Can you work these out from the model? Positions are in its coordinate system, mm. Face numbers are marked on the shaded views. A direction names the side the tool comes from. Coordinates: 2 decimals unless noted, no trailing zeros. Order: outer loops, then holes, each group sorted by start corner. A loop starts at its lowest first (then second) coordinate and runs counter-clockwise, first axis right, second up. Notation, with made-up numbers: (27.5, 35.5) - (54.5, 35.5) arc R12 cw to (54.5, 56.5) - close; hole circle Ø10 at (-31, 75.25). An arc over 180 degrees is marked (long way). Use a Markdown table: item, result. Add a question column.
(1) I want a section at A-A (z = -11). List the corners of the cut face in (x, y) for me.
(2) If I drill on L1, parallel to Z at x = -0.75, y = 3; L2, parallel to X at y = 3, z = -1; L3, parallel to Z at x = 5.5, y = 9, over which ranges is the centre line in solid material (lowest first)? Write a range as [from, to].
(3) On a 3-axis mill with a long thin cutter (end or side, diameter ignored), from which of +Z, -Z, +X, -X, +Y, -Y can I reach the whole of each face in a straight line? I mean the marked faces 4, 5 and 6. Say none if no direction works.
(4) For pin 1 Ø4 at (y, z) = (-28, 11.5) entering from -X; pin 2 Ø4 at (y, z) = (-28, 16) entering from +X; pin 3 Ø1 at (x, z) = (3, 16.5) entering from +Y, each with a flat end and sliding along its axis, tell me the tip position at first contact or that it passes through.
(5) We'd pull the mould along Z, two halves only. Please class the marked faces 1, 2 and 3: pulls with the +Z half, pulls with the -Z half, needs draft (parallel to the pull), parting line crosses it, or undercut.
```python
from build123d import *

# Parameters (mm, degrees)
SKETCH1_W           = 10
SKETCH1_H           = 10
BOSS_EXTRUDE1_DEPTH = 10
SKETCH2_R           = 5
BOSS_EXTRUDE2_DEPTH = 10
SKETCH4_R           = 4
BOSS_EXTRUDE3_DEPTH = 40
BOSS_EXTRUDE4_DEPTH = 10
CUT_EXTRUDE1_DEPTH  = 10
FILLET2_R           = 5
SKETCH7_W           = 14
SKETCH7_H           = 14
BOSS_EXTRUDE5_DEPTH = 2


with BuildPart() as part:
    # Sketch1 → Boss-Extrude1 (new body)
    with BuildSketch(Plane(origin=(0, 0, 0), x_dir=(1, 0, 0), z_dir=(0, 1, 0))):
        with Locations((5, 5)):
            Rectangle(SKETCH1_W, SKETCH1_H)
    extrude(amount=BOSS_EXTRUDE1_DEPTH)

    # Sketch2 → Boss-Extrude2 (add)
    with BuildSketch(Plane(origin=(0, 0, -10), x_dir=(-1, 0, 0), z_dir=(0, 0, -1))):
        with Locations((-5, 5)):
            Circle(SKETCH2_R)
    extrude(amount=BOSS_EXTRUDE2_DEPTH)

    # Sketch4 → Boss-Extrude3 (add)
    with BuildSketch(Plane(origin=(9.62e-07, 9.026239035, -5.211301537), x_dir=(0, -0.49999999999999467, -0.8660254037844417), z_dir=(-9.225892847871432e-08, -0.8660254037844382, 0.4999999999999926))):
        with Locations(Location((2.59569937, 4.999999038, 0), (0, 0, 229.539411428))):
            Circle(SKETCH4_R)
    extrude(amount=BOSS_EXTRUDE3_DEPTH)

    # Sketch5 → Boss-Extrude4 (add)
    with BuildSketch(Plane(origin=(0, 0, 0), x_dir=(0, 0, -1), z_dir=(1, 0, 0))):
        with BuildLine():
            Line((-16.004858714, -24.912627201), (-9.076655484, -28.912627201))
            ThreePointArc((-9.076655484, -28.912627201), (-6.076655484, -34.108779624), (-9.076655484, -39.304932046))
            Line((-9.076655484, -39.304932046), (-12.71063008, -37.206855835))
            Line((-12.71063008, -37.206855835), (-10.21063008, -32.876728816))
            Line((-10.21063008, -32.876728816), (-18.870884118, -27.876728816))
            Line((-18.870884118, -27.876728816), (-21.370884118, -32.206855835))
            Line((-21.370884118, -32.206855835), (-25.004858714, -30.108779624))
            ThreePointArc((-25.004858714, -30.108779624), (-22.004858714, -24.912627201), (-16.004858714, -24.912627201))
        make_face()
    extrude(amount=BOSS_EXTRUDE4_DEPTH)

    # Sketch6 → Cut-Extrude1 (cut)
    with BuildSketch(Plane(origin=(0, -33.40900615, 19.288698694), x_dir=(-1, 0, 0), z_dir=(0, -0.8660254037844403, 0.4999999999999971))):
        with BuildLine():
            Line((0, -7.40430063), (0, -2.40430063))
            ThreePointArc((0, -2.40430063), (-1.464466094, -5.939834536), (-5, -7.40430063))
            Line((-5, -7.40430063), (0, -7.40430063))
        make_face()
        with BuildLine():
            Line((-10, -7.40430063), (-5, -7.40430063))
            ThreePointArc((-5, -7.40430063), (-8.535533906, -5.939834536), (-10, -2.40430063))
            Line((-10, -2.40430063), (-10, -7.40430063))
        make_face()
        with BuildLine():
            ThreePointArc((-7.718879336, 11.791851793), (-6.417610293, 12.390527944), (-5, 12.59569937))
            Line((-5, 12.59569937), (-10, 12.59569937))
            Line((-10, 12.59569937), (-10, 11.791851793))
            Line((-10, 11.791851793), (-7.718879336, 11.791851793))
        make_face()
        with BuildLine():
            ThreePointArc((-10, 7.59569937), (-9.392857651, 9.983753318), (-7.718879336, 11.791851793))
            Line((-7.718879336, 11.791851793), (-10, 11.791851793))
            Line((-10, 11.791851793), (-10, 7.59569937))
        make_face()
        with BuildLine():
            Line((-2.281120664, 11.791851793), (0, 11.791851793))
            Line((0, 11.791851793), (0, 12.59569937))
            Line((0, 12.59569937), (-5, 12.59569937))
            ThreePointArc((-5, 12.59569937), (-3.582389707, 12.390527944), (-2.281120664, 11.791851793))
        make_face()
        with BuildLine():
            ThreePointArc((-2.281120664, 11.791851793), (-0.607142349, 9.983753318), (0, 7.59569937))
            Line((0, 7.59569937), (0, 11.791851793))
            Line((0, 11.791851793), (-2.281120664, 11.791851793))
        make_face()
    extrude(amount=-CUT_EXTRUDE1_DEPTH, mode=Mode.SUBTRACT)

    # Fillet2
    fillet2_edges = [part.edges().sort_by_distance(p)[0] for p in [
        (5, 10, 0),
    ]]
    fillet(fillet2_edges, radius=FILLET2_R)

    # Sketch7 → Boss-Extrude5 (add)
    with BuildSketch(Plane(origin=(0, 0, -10), x_dir=(-1, 0, 0), z_dir=(0, 0, -1))):
        with Locations((-5, 5)):
            Rectangle(SKETCH7_W, SKETCH7_H)
    extrude(amount=-BOSS_EXTRUDE5_DEPTH)


solid = part.part
```
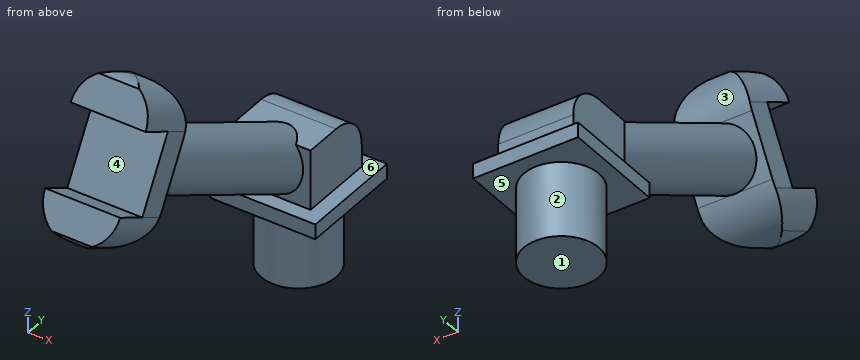
Answers follow:
| question | item | result |
|---|---|---|
| 1 | outline | circle Ø10 at (5, 5) |
| 2 | L1 | z = [-10, -8] |
| 2 | L2 | x = [0, 10] |
| 2 | L3 | z = [-20, -2] |
| 3 | face 4 | +X, -X |
| 3 | face 5 | -Z |
| 3 | face 6 | none |
| 4 | pin 1 | stops at x = 0 |
| 4 | pin 2 | stops at x = 10 |
| 4 | pin 3 | stops at y = -24.45 |
| 5 | face 1 | pulls with the -Z half |
| 5 | face 2 | needs draft |
| 5 | face 3 | undercut |
